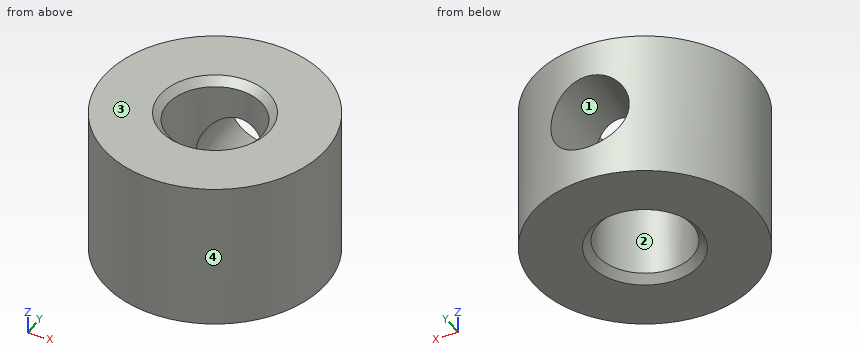
from build123d import *

# Parameters (mm, degrees)
F0_R     = 9.525
F1_DEPTH = 6.35
F2_R     = 4.05765
F3_DEPTH = 12.7
F4_R     = 2.85
F5_DEPTH = 9.526
F5_TAPER = -3
F6_SIZE  = 0.635


with BuildPart() as f1:
    # F0 (on Top) → F1 (new body, symmetric)
    with BuildSketch(Plane.XY):
        Circle(F0_R)
    extrude(amount=F1_DEPTH, both=True)

    # F2 (on Top) → F3 (cut, symmetric)
    with BuildSketch(Plane.XY):
        Circle(F2_R)
    extrude(amount=F3_DEPTH, both=True, mode=Mode.SUBTRACT)

    # F4 (on Front) → F5 (cut, through all)
    with BuildSketch(Plane.XZ):
        Circle(F4_R)
    extrude(amount=-F5_DEPTH, taper=F5_TAPER, mode=Mode.SUBTRACT)

    # F6
    f6_edges = [f1.edges().sort_by_distance(p)[0] for p in [
        (-4.05765, 0, -6.35),
        (-4.05765, 0, 6.35),
    ]]
    chamfer(f6_edges, length=F6_SIZE)


solid = f1.part
Read the model definition and answer for the solid it produces. Units are mm, in the model's axes. Face numbers are marked on the shaded views. Coordinates: 2 decimals unless noted, no trailing zeros. Loops run counter-clockwise (first coordinate to the right, second up) from the corner with the lowest first, then second, coordinate; pieces in that order, holes last. Notation, with made-up numbers: (34, 21) - (54, 21) arc R16 cw to (54, 44) - close; hole circle Ø1 at (30.25, -19.75). An arc over 180 degrees is marked (long way). Answer in a Markdown table with one row per item.
Q1. The mould has two halves that part along X. Classify the marked faces 1, 2, 3 and 4: pulls with the +X half, pulls with the -X half, needs draft (parallel to the pull), parting line crosses it, or undercut.
Here are the results:
| item | result |
|---|---|
| face 1 | undercut |
| face 2 | undercut |
| face 3 | needs draft |
| face 4 | parting line crosses it |
Q2. Straight lines are drawn through the part: line 1 along Y through (x, z) = (0, -0.5) (3 decimals); line 2 along X through (y, z) = (6, 0.75); line 3 along X through (y, z) = (-2.25, 4). For each, find the intervals that lie inside material, in ascending order. Write a range as [from, to].
Here are the results:
| item | result |
|---|---|
| line 1 | y = [-9.525, -4.058] |
| line 2 | x = [-7.4, -3.07], [3.07, 7.4] |
| line 3 | x = [-9.26, -3.38], [3.38, 9.26] |
Q3. Find section A-A on y = 0. Write down the section's boundary in (x, z) (3 decimals), plus the area to 3 significant figures.
Here are the results:
| item | result |
|---|---|
| outline | (-9.525, -6.35) - (-4.693, -6.35) - (-4.058, -5.715) - (-4.058, 5.715) - (-4.693, 6.35) - (-9.525, 6.35) - close; (4.058, -5.715) - (4.693, -6.35) - (9.525, -6.35) - (9.525, 6.35) - (4.693, 6.35) - (4.058, 5.715) - close |
| area | 138 mm^2 |
Q4. Find section C-C on z = -4. Write down the section's boundary in (x, y) (3 decimals), plus the area to 3 significant figures.
Here are the results:
| item | result |
|---|---|
| outline | circle Ø19.05 at (0, 0); hole circle Ø8.115 at (0, 0) |
| area | 233 mm^2 |
Q5. Find section B-B on x = 0. Write down the section's boundary in (y, z) (3 decimals), plus the area to 3 significant figures.
Here are the results:
| item | result |
|---|---|
| outline | (-9.525, -6.35) - (-4.693, -6.35) - (-4.058, -5.715) - (-4.058, 5.715) - (-4.693, 6.35) - (-9.525, 6.35) - close; (4.058, -5.715) - (4.693, -6.35) - (9.525, -6.35) - (9.525, -3.349) - (4.058, -3.063) - close; (4.058, 3.063) - (9.525, 3.349) - (9.525, 6.35) - (4.693, 6.35) - (4.058, 5.715) - close |
| area | 103 mm^2 |
Q6. Find section D-D on x = 7.25. Write down the section's boundary in (y, z), plus the area to 3 significant figures.
Here are the results:
| item | result |
|---|---|
| outline | (-6.18, -6.35) - (6.18, -6.35) - (6.18, 6.35) - (-6.18, 6.35) - close |
| area | 157 mm^2 |
Q7. Given P1, Ø1.5, axis at x = 6.5, z = 3, coming from the -Y side; P2, Ø7.5, axis at x = 0, y = 0, coming from the +Z side; P3, Ø5, axis at x = -7, z = -5, coming from the +Y side (3 decimals); P4, Ø1.5, axis at x = -5, z = 1.5, coming from the +Y side, each flat-ended and moving along its own axis, determine where each tip first touches the part or whether it passes through.
Here are the results:
| item | result |
|---|---|
| P1 | stops at y = -7.59 |
| P2 | passes through |
| P3 | stops at y = 8.395 |
| P4 | stops at y = 8.52 |
